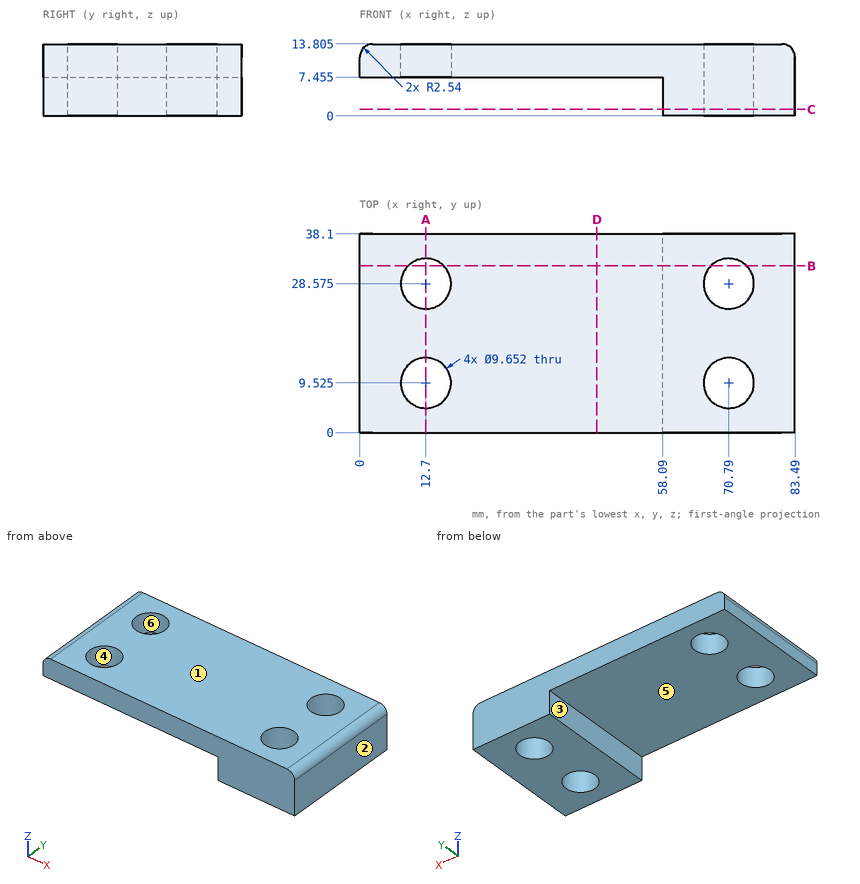
Source: three-view drawing plus pictorial views. Frame: mm from the lowest corner of the part. A direction names the side the tool comes from. Coordinates: 2 decimals unless noted, no trailing zeros. Order: outer loops, then holes, each group sorted by start corner. A loop starts at its lowest first (then second) coordinate and runs counter-clockwise, first axis right, second up. Notation, with made-up numbers: M -38.5,40 L -28.5,40 A11 cw -28.5,53 Z; hole C -32,83 d9. An arc over 180 degrees is marked long. One line per question, with ' | ' between items. Start each with the question number.
Item 1: Set-up query: the marked faces 5 and 6. Return all of +Z, -Z, +X, -X, +Y, -Y with unobstructed straight access to the full face (end or side cutting, diameter ignored); none if empty.
Item 2: Cut plane A-A, the plane x = 12.7. Return the cut outline in (y, z) (1 decimal), then the cut area to 3 significant figures.
Item 3: Cut plane B-B, the plane y = 32. Count the separate pieces of the cut face and the enclosed holes in it, then the cut area to 3 significant figures.
Item 4: Cut plane D-D, the plane x = 45.5. Return the cut outline in (y, z) (1 decimal).
Item 5: Cut plane C-C, the plane z = 1.25. Return the cut outline in (x, y) (1 decimal), then the cut area to 3 significant figures.
Item 6: Ray query, probe 1 along Y at (x, z) = (12.7, 11.5); probe 2 along X at (y, z) = (28.5, 10.5) (1 decimal). Return the intervals inside material, ascending. Write a range as [from, to].
Item 7: Draft query along X for the marked faces 1, 2, 3 and 4. Return one class per face: released by +X, released by -X, zero draft, split by the parting line, or undercut.
Item 8: Pin query (flat end, axial travel): pin 1 Ø19 at (x, y) = (23, 22) entering from -Z (3 decimals); pin 2 Ø6 at (x, y) = (70.79, 9.52) entering from +Z; pin 3 Ø15.5 at (x, y) = (70.79, 28.58) entering from +Z (3 decimals); pin 4 Ø6 at (y, z) = (16, 3.5) entering from -X. Return the tip coordinate at first contact, or that it passes through.
A:
1) face 5: -Z, -X, +Y, -Y | face 6: +Z, -Z
2) outline: M 0,7.5 L 4.7,7.5 L 4.7,13.8 L 0,13.8 Z; M 14.4,7.5 L 23.7,7.5 L 23.7,13.8 L 14.4,13.8 Z; M 33.4,7.5 L 38.1,7.5 L 38.1,13.8 L 33.4,13.8 Z | area: 119 mm2
3) separate pieces: 3 | enclosed holes: 0 | area: 580 mm2
4) outline: M 0,7.5 L 38.1,7.5 L 38.1,13.8 L 0,13.8 Z
5) outline: M 58.1,0 L 83.5,0 L 83.5,38.1 L 58.1,38.1 Z; hole C 70.8,9.5 d9.7; hole C 70.8,28.6 d9.7 | area: 821 mm2
6) probe 1: y = [0, 4.7], [14.35, 23.75], [33.4, 38.1] | probe 2: x = [0, 7.9], [17.5, 66], [75.6, 83.5]
7) face 1: zero draft | face 2: released by +X | face 3: released by -X | face 4: undercut
8) pin 1: stops at z = 7.455 | pin 2: passes through | pin 3: stops at z = 13.805 | pin 4: stops at x = 58.09
